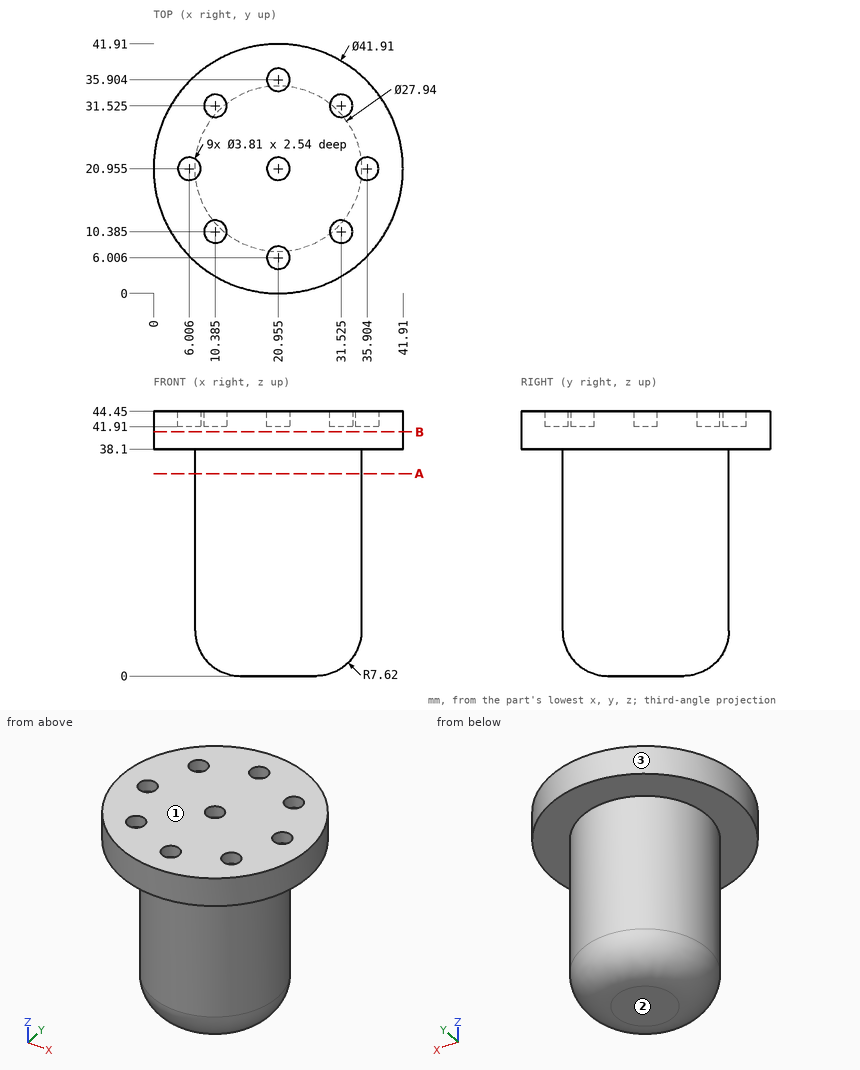
Part print with two shaded views. Sizes in mm from the minimum x, y, z corner. Round coordinates to 2 decimals unless told otherwise and drop trailing zeros. Order: outer loops, then holes, each group sorted by start corner. A loop starts at its lowest first (then second) coordinate and runs counter-clockwise, first axis right, second up. Notation, with made-up numbers: M 23.5,31 L 39.5,31 A20 ccw 39.5,70 Z; hole C -28,60 d5. An arc over 180 degrees is marked long. Use CSV: the item, a comma, the result in double quotes.
Item 1: Saw through at B-B (z = 41). List the corners of the cut face in (x, y) (1 decimal).
Worked answers:
outline,"C 21,21 d41.9"
Item 2: Pin check, flat tips, straight feed: pin 1 (6 mm diameter, centred on x = 27.5, z = 28, fed in from -Y); pin 2 (8 mm diameter, centred on x = 32.5, y = 27.5, fed in from -Z); pin 3 (8 mm diameter, centred on y = 35, z = 23.5, fed in from -X) (1 decimal). Stop position of each tip, or through.
Worked answers:
pin 1,"y = 7.44"
pin 2,"z = 0.58"
pin 3,"x = 11.2"
Item 3: Saw through at A-A (z = 34). List the corners of the cut face in (x, y) (1 decimal), plus the area to 3 significant figures.
Worked answers:
outline,"C 21,21 d27.9"
area,"613 mm²"
Item 4: Probe probe 1 along Z at (x, y) = (32, 12); probe 2 along Z at (x, y) = (33, 9); probe 3 along X at (y, z) = (8.5, 39.5) (1 decimal). List the from-to ranges inside material, lowest first.
Worked answers:
probe 1,"38.1 to 41.91"
probe 2,"38.1 to 44.45"
probe 3,"4.1 to 37.8"
Item 5: Pull direction Z, two halves, no side cores. Call the marked faces 1, 2 and 3: released by +Z, released by -Z, zero draft, split by the parting line, or undercut.
Worked answers:
face 1,"released by +Z"
face 2,"released by -Z"
face 3,"zero draft"
